from build123d import *

# Parameters (mm, degrees)
ESQUISSE1_W                  = 89
ESQUISSE1_H                  = 89
MAIN_EXTRUSION_DEPTH         = 18
ESQUISSE2_R                  = 2
FIXATION_HOLE_DEPTH          = 19
ESQUISSE3_W                  = 9
ESQUISSE3_H                  = 9
FIXATION_SQUARE_DEPTH        = 15
CPU_RJ11_DEPTH               = 16
ESQUISSE5_W                  = 10
ESQUISSE5_H                  = 71
ENL_V_MAT_EXTRU_4_DEPTH      = 19
ESQUISSE6_W                  = 67
ESQUISSE6_H                  = 14
ESQUISSE6_W_2                = 16
ESQUISSE6_H_2                = 11
ESQUISSE6_W_3                = 29
HE10_CONNECTORS_DEPTH        = 8
ESQUISSE7_W                  = 8
ESQUISSE7_H                  = 14
ESQUISSE7_H_2                = 10
HE10_CONNECTORS_TOP_DEPTH    = 81
ESQUISSE9_W                  = 10
ESQUISSE9_H                  = 10
ENL_V_MAT_EXTRU_7_DEPTH      = 1
ENL_V_MAT_EXTRU_7_DEPTH_BACK = 19


with BuildPart() as part:
    # Esquisse1 → Main Extrusion (new body)
    with BuildSketch(Plane.XY):
        Rectangle(ESQUISSE1_W, ESQUISSE1_H)
    extrude(amount=MAIN_EXTRUSION_DEPTH)

    # Esquisse2 → Fixation Hole (cut, through all)
    with BuildSketch(Plane.XY.offset(18)):
        with Locations((-39.5, 39.5)):
            Circle(ESQUISSE2_R)
        with Locations((39.5, 39.5)):
            Circle(ESQUISSE2_R)
        with Locations((39.5, -39.5)):
            Circle(ESQUISSE2_R)
        with Locations((-39.5, -39.5)):
            Circle(ESQUISSE2_R)
    extrude(amount=-FIXATION_HOLE_DEPTH, mode=Mode.SUBTRACT)

    # Esquisse3 → Fixation Square (cut)
    with BuildSketch(Plane.XY.offset(18)):
        with Locations((-40, 40)):
            Rectangle(ESQUISSE3_W, ESQUISSE3_H)
        with Locations((-40, -40)):
            Rectangle(ESQUISSE3_W, ESQUISSE3_H)
        with Locations((40, -40)):
            Rectangle(ESQUISSE3_W, ESQUISSE3_H)
        with Locations((40, 40)):
            Rectangle(ESQUISSE3_W, ESQUISSE3_H)
    extrude(amount=-FIXATION_SQUARE_DEPTH, mode=Mode.SUBTRACT)

    # Esquisse4 → CPU + RJ11 (cut)
    with BuildSketch(Plane(origin=(0, 0, 0), x_dir=(-1, 0, 0), z_dir=(0, 0, -1))):
        Polygon((-32.5, -32.5), (-15.5, -32.5), (-15.5, -44.5), (2.5, -44.5), (2.5, -32.5), (32.5, -32.5), (32.5, 28.5), (-32.5, 28.5), align=None)
    extrude(amount=-CPU_RJ11_DEPTH, mode=Mode.SUBTRACT)

    # Esquisse5 → Enlèv. mat.-Extru.4 (cut, through all)
    with BuildSketch(Plane.XY.offset(18)):
        with Locations((-39.5, 0)):
            Rectangle(ESQUISSE5_W, ESQUISSE5_H)
        with Locations((39.5, 0)):
            Rectangle(ESQUISSE5_W, ESQUISSE5_H)
    extrude(amount=-ENL_V_MAT_EXTRU_4_DEPTH, mode=Mode.SUBTRACT)

    # Esquisse6 → HE10 Connectors (cut)
    with BuildSketch(Plane(origin=(0, 0, 0), x_dir=(-1, 0, 0), z_dir=(0, 0, -1))):
        with Locations((0, 37.5)):
            Rectangle(ESQUISSE6_W, ESQUISSE6_H)
        with Locations((-25.5, -39)):
            Rectangle(ESQUISSE6_W_2, ESQUISSE6_H_2)
        with Locations((19, -39)):
            Rectangle(ESQUISSE6_W_3, ESQUISSE6_H_2)
    extrude(amount=-HE10_CONNECTORS_DEPTH, mode=Mode.SUBTRACT)

    # Esquisse7 → HE10 Connectors Top (cut, through all)
    with BuildSketch(Plane.ZY.offset(35.5)):
        with Locations((14, 37.5)):
            Rectangle(ESQUISSE7_W, ESQUISSE7_H)
        with Locations((14, -39.5)):
            Rectangle(ESQUISSE7_W, ESQUISSE7_H_2)
    extrude(amount=-HE10_CONNECTORS_TOP_DEPTH, mode=Mode.SUBTRACT)

    # Esquisse9 → Enlèv. mat.-Extru.7 (cut, two sides)
    with BuildSketch(Plane.XY.offset(18)) as enl_v_mat_extru_7_sk:
        with Locations((-4.5, -31.5)):
            Rectangle(ESQUISSE9_W, ESQUISSE9_H)
    extrude(amount=ENL_V_MAT_EXTRU_7_DEPTH, mode=Mode.SUBTRACT)
    extrude(enl_v_mat_extru_7_sk.sketch, amount=-ENL_V_MAT_EXTRU_7_DEPTH_BACK, mode=Mode.SUBTRACT)


solid = part.part
The model under review builds one solid part; all positions refer to its coordinate system, in mm. A direction names the side the tool comes from. Give positions to 0.01 mm unless a question says otherwise; leave off trailing zeros. Loops run counter-clockwise (first coordinate to the right, second up) from the corner with the lowest first, then second, coordinate; pieces in that order, holes last. Notation, with made-up numbers: (45, 17.5) -> (90, 17.5) arc R32 ccw to (90, 48.5) -> close; hole circle Ø10 at (-3.75, 41.25). An arc over 180 degrees is marked (long way). Answer as a JSON object with one key per item and string values. Group by question number.
Q1. Tool access review of faces 1 (the flat face through (-34.5, 0, 9)), 2 (the flat face through (35.5, 40, 7)), 3 (the flat face through (-35.5, -40, 7)): name each direction out of +Z, -Z, +X, -X, +Y, -Y from which nothing blocks a thin tool from reaching the whole face with its end or side.
Q2. Insertion check: pin 1 (5 mm diameter, centred on x = 24.5, y = -39.5, fed in from +Z); pin 2 (3.5 mm diameter, centred on x = -7.5, z = 4, fed in from +Y); pin 3 (1.5 mm diameter, centred on y = -21, z = 15.5, fed in from -X); pin 4 (10 mm diameter, centred on x = -9.5, z = 5, fed in from -Y). Each pin has a flat end and moves straight along its axis. Give the tip position at first contact, or say it passes through.
Q3. Take a section at B-B (y = 39.5). Write out the cut boundary in (x, z).
Q4. Wall thickness on line 1 along Y through (x, z) = (39.5, 2.05); line 2 along Y through (x, z) = (-7.5, 9.5); line 3 along X through (y, z) = (-18, 6.5): over which ranges is each line inside the solid? List them lowest first.
Q5. Draft analysis for pull direction Y (two halves, no side actions). For faces 4 (the flat face through (-0.2, 44.5, 8.3)), 5 (the flat face through (21, -34.5, 15)), 6 (the flat face through (-19, -40, 10)), 7 (the flat face through (-9.5, -33, 12)), state which applies: pulls with the +Y half, pulls with the -Y half, needs draft (parallel to the pull), parting line crosses it, or undercut.
Q6. Take a section at D-D (y = -39.5). Write out the cut boundary in (x, z).
Q7. Take a section at A-A (x = -7). Write out the cut boundary in (y, z), plus the area to 3 significant figures.
Answer below:
{
 "1": {"face 1": "+Z, -Z, -X", "face 2": "+Z, +X, +Y, -Y", "face 3": "+Z, -X, +Y, -Y"},
 "2": {"pin 1": "stops at z = 10", "pin 2": "stops at y = 30.5", "pin 3": "stops at x = -34.5", "pin 4": "stops at y = -44.5"},
 "3": {"outline": "(-44.5, 0) -> (-41.5, 0) -> (-41.5, 3) -> (-44.5, 3) -> close; (-37.5, 0) -> (-33.5, 0) -> (-33.5, 8) -> (33.5, 8) -> (33.5, 0) -> (37.5, 0) -> (37.5, 3) -> (35.5, 3) -> (35.5, 10) -> (-35.5, 10) -> (-35.5, 3) -> (-37.5, 3) -> close; (41.5, 0) -> (44.5, 0) -> (44.5, 3) -> (41.5, 3) -> close"},
 "4": {"line 1": "y = -44.5 to -41.5, -37.5 to -35.5, 35.5 to 37.5, 41.5 to 44.5", "line 2": "y = -44.5 to -36.5, 28.5 to 44.5", "line 3": "x = -34.5 to -32.5, 32.5 to 34.5"},
 "5": {"face 4": "pulls with the +Y half", "face 5": "pulls with the -Y half", "face 6": "needs draft", "face 7": "undercut"},
 "6": {"outline": "(-44.5, 0) -> (-41.5, 0) -> (-41.5, 3) -> (-44.5, 3) -> close; (-37.5, 0) -> (-33.5, 0) -> (-33.5, 8) -> (-4.5, 8) -> (-4.5, 0) -> (-2.5, 0) -> (-2.5, 10) -> (-35.5, 10) -> (-35.5, 3) -> (-37.5, 3) -> close; (15.5, 0) -> (17.5, 0) -> (17.5, 8) -> (33.5, 8) -> (33.5, 0) -> (37.5, 0) -> (37.5, 3) -> (35.5, 3) -> (35.5, 10) -> (15.5, 10) -> close; (41.5, 0) -> (44.5, 0) -> (44.5, 3) -> (41.5, 3) -> close"},
 "7": {"outline": "(-44.5, 8) -> (-36.5, 8) -> (-36.5, 10) -> (-44.5, 10) -> close; (-26.5, 16) -> (28.5, 16) -> (28.5, 0) -> (30.5, 0) -> (30.5, 8) -> (44.5, 8) -> (44.5, 10) -> (30.5, 10) -> (30.5, 18) -> (-26.5, 18) -> close", "area": "190 mm2"}
}
